```python
from build123d import *

# Parameters (mm, degrees)
F0_W     = 200
F0_H     = 200
F0_R     = 8.5
F1_DEPTH = 20
F2_W     = 265.768706
F2_H     = 235.001818
F3_DEPTH = 3


with BuildPart() as f1:
    # F0 (on Top) → F1 (new body)
    with BuildSketch(Plane.XY):
        Rectangle(F0_W, F0_H)
        with Locations((-85, -85)):
            Circle(F0_R, mode=Mode.SUBTRACT)
        with Locations((85, -85)):
            Circle(F0_R, mode=Mode.SUBTRACT)
        with Locations((-85, 85)):
            Circle(F0_R, mode=Mode.SUBTRACT)
        with Locations((85, 85)):
            Circle(F0_R, mode=Mode.SUBTRACT)
    extrude(amount=F1_DEPTH)

    # F2 (on face) → F3 (cut)
    with BuildSketch(Plane(origin=(0, 0, 0), x_dir=(1, 0, 0), z_dir=(0, 0, -1))):
        Rectangle(F2_W, F2_H)
    extrude(amount=-F3_DEPTH, mode=Mode.SUBTRACT)


solid = f1.part
```
Verification items for the finished model (mm, model axes). Coordinates: 2 decimals unless noted, no trailing zeros. Loops run counter-clockwise (first coordinate to the right, second up) from the corner with the lowest first, then second, coordinate; pieces in that order, holes last. Notation, with made-up numbers: (-3, 20) - (19, 20) arc R9 ccw to (19, 36) - close; hole circle Ø3 at (-34.5, -25.75). An arc over 180 degrees is marked (long way). Return JSON: item names as keys, results as strings.
1. Mould release check, pull along Y, two halves, no side actions. Record for faces 1 (the cylindrical face through (76.51, -84.63, 11.38)), 2 (the flat face through (-1, 100, 11)), 3 (the flat face through (-100, -1, 11)): +Y half, -Y half, draft (parallel to the pull), parting line (faces both ways), or undercut.
Established:
{"face 1": "undercut", "face 2": "+Y half", "face 3": "draft"}
2. Section check C-C, the plane z = 14.25. Record the boundary of the cut face in (x, y), then the cut area to 3 significant figures.
Established:
{"outline": "(-100, -100) - (100, -100) - (100, 100) - (-100, 100) - close; hole circle Ø17 at (-85, -85); hole circle Ø17 at (-85, 85); hole circle Ø17 at (85, -85); hole circle Ø17 at (85, 85)", "area": "39,100 mm2"}
3. Section check A-A, the plane y = -85. Record the boundary of the cut face in (x, z), then the cut area to 3 significant figures.
Established:
{"outline": "(-100, 3) - (-93.5, 3) - (-93.5, 20) - (-100, 20) - close; (-76.5, 3) - (76.5, 3) - (76.5, 20) - (-76.5, 20) - close; (93.5, 3) - (100, 3) - (100, 20) - (93.5, 20) - close", "area": "2,820 mm2"}
4. Thickness scan on L1, parallel to X at y = 85, z = 16.5; L2, parallel to X at y = -88.5, z = 13. Record the ranges inside material, lowest first.
Established:
{"L1": "x = -100 to -93.5, -76.5 to 76.5, 93.5 to 100", "L2": "x = -100 to -92.75, -77.25 to 77.25, 92.75 to 100"}
